Geometry check sheet. Reference: the model listing, model coordinates, mm. Coordinates: 2 decimals unless noted, no trailing zeros. Order: outer loops, then holes, each group sorted by start corner. A loop starts at its lowest first (then second) coordinate and runs counter-clockwise, first axis right, second up. Notation, with made-up numbers: (21, 80) - (69, 80) arc R20 cw to (69, 112) - close; hole circle Ø4 at (46.25, -31.75). An arc over 180 degrees is marked (long way). Return JSON: item names as keys, results as strings. Group by question number.
Item 1: Scan lines: probe 1 along X at (y, z) = (0, 1.45); probe 2 along Y at (x, z) = (30, 2.05); probe 3 along X at (y, z) = (0.75, 2.35). Record each from-to range of solid material in increasing order.
Item 2: Gauge pin test, flat end, axial feed: pin 1 (1.8 mm diameter, centred on x = 31, y = 0, fed in from -Z). Record the tip position at first contact, or that the pin passes through.
Item 3: Section check C-C on y = 0. Enter the section's corners in (x, z).
Item 4: Section check A-A on z = 2. Enter the section's corners in (x, y).
Item 5: Section check B-B on x = 30. Enter the section's corners in (y, z).
Solid Edge part; units mm, degrees
sketch "Sketch1" plane through (0, 0, 0) normal (0, 0, 1) x (1, 0, 0)
  line L0 (-40, -15) -> (40, -15)
  line L1 (40, -15) -> (40, 15)
  line L2 (40, 15) -> (-40, 15)
  line L3 (-40, 15) -> (-40, -15)
extrude "Protrusion1" add sketch "Sketch1" along normal blind 4
hole "Hole_1" at (30, 0, 0) direction (0, 0, 1) diameter 6 depth 3
hole "Hole1" at (-30, 0, 0) direction (0, 0, 1) diameter 6 depth 3
fillet "Round_1" radius 5 4 edges at (-40, 15, 2) (-40, -15, 2) (40, -15, 2) (40, 15, 2)
chamfer "Chamfer_1" distance 1 angle 45 8 edges at (-40, 0, 4) (-38.5355, -13.5355, 4) (0, -15, 4) (38.5355, -13.5355, 4) (40, 0, 4) (38.5355, 13.5355, 4) (0, 15, 4) (-38.5355, 13.5355, 4)
properties material "Bronze, 90%"
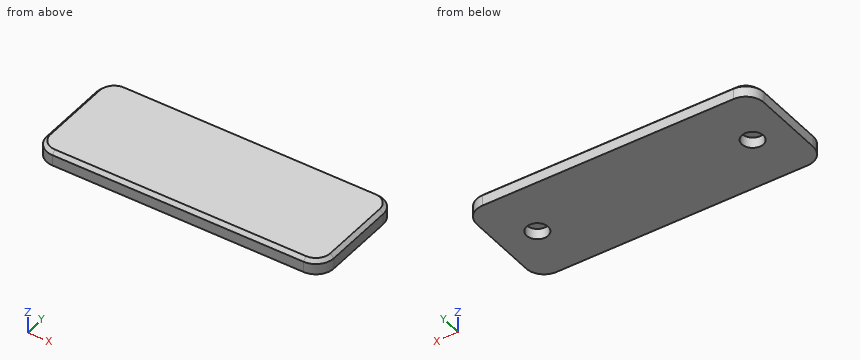
Computed:
{
 "1": {"probe 1": "x = -40 to -33, -27 to 27, 33 to 40", "probe 2": "y = -15 to -3, 3 to 15", "probe 3": "x = -40 to -32.9, -27.1 to 27.1, 32.9 to 40"},
 "2": {"pin 1": "stops at z = 3"},
 "3": {"outline": "(-40, 0) - (-33, 0) - (-33, 3) - (-27, 3) - (-27, 0) - (27, 0) - (27, 3) - (33, 3) - (33, 0) - (40, 0) - (40, 3) - (39, 4) - (-39, 4) - (-40, 3) - close"},
 "4": {"outline": "(-40, -10) arc R5 ccw to (-35, -15) - (35, -15) arc R5 ccw to (40, -10) - (40, 10) arc R5 ccw to (35, 15) - (-35, 15) arc R5 ccw to (-40, 10) - close; hole circle Ø6 at (-30, 0); hole circle Ø6 at (30, 0)"},
 "5": {"outline": "(-15, 0) - (-3, 0) - (-3, 3) - (3, 3) - (3, 0) - (15, 0) - (15, 3) - (14, 4) - (-14, 4) - (-15, 3) - close"}
}
